Input: part model. Units: mm. Frame: model coordinates. A direction names the side the tool comes from. Coordinates: 2 decimals unless noted, no trailing zeros. Write each loop counter-clockwise with the first axis right and the second up, starting at its lowest first coordinate (ties: lowest second). Pieces come first, ordered by that corner, then holes.
from build123d import *

# Parameters (mm, degrees)
SKETCH1_W           = 114.3
SKETCH1_H           = 114.3
SKETCH1_W_2         = 101.6
SKETCH1_H_2         = 101.6
EXTRUDE_THIN1_DEPTH = 50.8
SKETCH3_W           = 114.3
SKETCH3_H           = 114.3
SKETCH3_W_2         = 101.6
SKETCH3_H_2         = 101.6
EXTRUDE_THIN2_DEPTH = 50.8
BOSS_EXTRUDE1_DEPTH = 114.3
SKETCH6_R           = 6.35
CUT_EXTRUDE1_DEPTH  = 224.426173489


with BuildPart() as part:
    # Sketch1 → Extrude-Thin1 (new body)
    with BuildSketch(Plane.XY):
        Rectangle(SKETCH1_W, SKETCH1_H)
        Rectangle(SKETCH1_W_2, SKETCH1_H_2, mode=Mode.SUBTRACT)
    extrude(amount=EXTRUDE_THIN1_DEPTH)

    # Sketch3 → Extrude-Thin2 (add)
    with BuildSketch(Plane(origin=(57.15, 0, 0), x_dir=(0, 0, -1), z_dir=(1, 0, 0))):
        with Locations((-101.6, 0)):
            Rectangle(SKETCH3_W, SKETCH3_H)
        with Locations((-101.6, 0)):
            Rectangle(SKETCH3_W_2, SKETCH3_H_2, mode=Mode.SUBTRACT)
    extrude(amount=EXTRUDE_THIN2_DEPTH)

    # Sketch4 → Boss-Extrude1 (add)
    with BuildSketch(Plane.ZY.offset(-57.15)):
        Polygon((50.8, -50.8), (50.8, -57.15), (158.75, -57.15), (158.75, 57.15), (50.8, 57.15), (50.8, 50.8), (152.4, 50.8), (152.4, -50.8), align=None)
    extrude(amount=BOSS_EXTRUDE1_DEPTH)

    # Sketch6 → Cut-Extrude1 (cut, through all)
    with BuildSketch(Plane(origin=(0, 57.15, 0), x_dir=(1, 0, 0), z_dir=(0, 1, 0))):
        with Locations(Location((0, -50.8, 0), (0, 0, 270))):
            Circle(SKETCH6_R)
    cut_extrude1 = extrude(amount=-CUT_EXTRUDE1_DEPTH, mode=Mode.SUBTRACT)

    # Mirror1: Cut-Extrude1 across plane
    add(cut_extrude1.mirror(Plane(origin=(50.8, 0, 50.8), x_dir=(-0.7071067811865477, 0, 0.7071067811865474), z_dir=(0.7071067811865476, 0, 0.7071067811865476))), mode=Mode.SUBTRACT)


solid = part.part
Item 1: Section query C-C, the plane y = 37.5. Return loops of the section in (x, z).
Item 2: Access query for faces 1 (the face through (27, -50.8, 77)), 2 (the face through (47.386, -53.931, 96.246)), 3 (the face through (50.8, -1, 25)), 4 (the face through (57.15, -1, 22)), 5 (the face through (-54, 1, 50.8)). Directions: +Z, -Z, +X, -X, +Y, -Y. A direction counts if a zero-diameter tool reaches every point of the face in a straight line with its end or side. Return the directions, or none.
Item 3: Material intervals for line 1 (Y direction, x = 77.5, z = 73.5); line 2 (X direction, y = 55, z = 50.8); line 3 (Z direction, x = 87, y = 27), sorted ascending.
Item 4: Section query A-A, the plane z = 83. Return loops of the section in (x, y), then the cut area to 3 significant figures.
Item 5: Pin query (flat end, axial travel): pin 1 Ø7.5 at (x, z) = (50.8, 101.6) entering from -Y; pin 2 Ø15 at (x, y) = (71, -9) entering from -Z; pin 3 Ø12 at (x, y) = (14, -23.5) entering from -Z. Return the tip coordinate at first contact, or that it passes through.
Item 6: Section query B-B, the plane x = 60. Return loops of the section in (y, z).
Item 7: Pull-direction query (Z, two-part tool) for faces 6 (the face through (79, 1, 50.8)), 7 (the face through (-50.8, -1, 25)), 8 (the face through (82, -1, 44.45)), 9 (the face through (27, -1, 158.75)); classes: released by +Z, released by -Z, zero draft, split by the parting line, or undercut.
Item 8: Section query D-D, the plane z = 101.6. Return loops of the section in (x, y).
The answers:
1. outline: (-57.15, 0) - (-50.8, 0) - (-50.8, 50.8) - (-57.15, 50.8) - close; (-57.15, 152.4) - (107.95, 152.4) - (107.95, 158.75) - (-57.15, 158.75) - close; (50.8, 0) - (57.15, 0) - (57.15, 44.45) - (107.95, 44.45) - (107.95, 50.8) - (50.8, 50.8) - close
2. face 1: none
2. face 2: +Y, -Y
2. face 3: -Z
2. face 4: -Z, +X, +Y, -Y
2. face 5: +X, -X
3. line 1: y = -57.15 to -50.8, 50.8 to 57.15
3. line 2: x = -57.15 to -6.35, 6.35 to 107.95
3. line 3: z = 44.45 to 50.8, 152.4 to 158.75
4. outline: (-57.15, -57.15) - (107.95, -57.15) - (107.95, -50.8) - (-57.15, -50.8) - close; (-57.15, 50.8) - (107.95, 50.8) - (107.95, 57.15) - (-57.15, 57.15) - close
4. area: 2,100 mm2
5. pin 1: passes through
5. pin 2: stops at z = 44.45
5. pin 3: stops at z = 152.4
6. outline: (-57.15, 44.45) - (57.15, 44.45) - (57.15, 158.75) - (-57.15, 158.75) - close; hole (-50.8, 50.8) - (50.8, 50.8) - (50.8, 152.4) - (-50.8, 152.4) - close
7. face 6: undercut
7. face 7: zero draft
7. face 8: released by -Z
7. face 9: released by +Z
8. outline: (-57.15, -57.15) - (44.45, -57.15) - (44.45, -50.8) - (-57.15, -50.8) - close; (-57.15, 50.8) - (44.45, 50.8) - (44.45, 57.15) - (-57.15, 57.15) - close; (57.15, -57.15) - (107.95, -57.15) - (107.95, -50.8) - (57.15, -50.8) - close; (57.15, 50.8) - (107.95, 50.8) - (107.95, 57.15) - (57.15, 57.15) - close
